Autodesk Inventor part; units mm, degrees
ref_plane "YZ Plane" through (0, 0, 0) normal (1, 0, 0) x (0, 1, 0)
ref_plane "XZ Plane" through (0, 0, 0) normal (0, 1, 0) x (-1, 0, 0)
ref_plane "XY Plane" through (0, 0, 0) normal (0, 0, 1) x (1, 0, 0)
sketch "Sketch1" plane through (0, 0, 0) normal (0, 0, 1) x (1, 0, 0)
  line L0 (38.1, -12.7) -> (-38.1, -12.7)
  line L1 (-38.1, -12.7) -> (-38.1, 12.7)
  line L2 (-38.1, 12.7) -> (38.1, 12.7)
  line L3 (38.1, 12.7) -> (38.1, -12.7)
  line L4 (38.1, -12.7) -> (-38.1, 12.7) construction
  line L5 (-38.1, -12.7) -> (38.1, 12.7) construction
  circle A0 centre (31.75, 6.35) radius 1.5875
  circle A1 centre (31.75, -6.35) radius 1.5875
  circle A2 centre (25.4, 6.35) radius 1.5875
  circle A3 centre (25.4, -6.35) radius 1.5875
  line L6 (-38.1, 12.7) -> (-63.5, 12.7)
  line L7 (-63.5, 12.7) -> (-63.5, -50.8)
  line L8 (-63.5, -50.8) -> (-38.1, -50.8)
  line L9 (-38.1, -50.8) -> (-38.1, 12.7)
  circle A4 centre (-38.1, -29.845) radius 17.145
  point P0 (0, 0)
  point P1 (-38.1, -46.99)
  dimension "d0" = 76.2
  dimension "d1" = 25.4
  dimension "d2" = 3.175
  dimension "d3" = 6.35
  dimension "d4" = 6.35
  dimension "d5" = 3.175
  dimension "d6" = 6.35
  dimension "d7" = 6.35
  dimension "d8" = 3.175
  dimension "d9" = 6.35
  dimension "d10" = 6.35
  dimension "d13" = 3.175
  dimension "d14" = 6.35
  dimension "d15" = 6.35
  dimension "d16" = 25.4
  dimension "d17" = 63.5
  dimension "d18" = 34.29
  dimension "d19" = 17.145
extrude "Extrusion1" add sketch "Sketch1" along normal blind 3.175 contours L0 L1 L2 L3 | A4 L9 L8 L7 L6 L1
fillet "Fillet1" radius 3.175 4 edges at (-38.1, -50.8, 1.5875) (-38.1, -46.99, 1.5875) (-63.5, -50.8, 1.5875) (-63.5, 12.7, 1.5875)
properties part number "Climb_Hooks_2"
Here's how the part is built. I have some questions about the finished solid (model axes, mm). Coordinates: 2 decimals unless noted, no trailing zeros. Order: outer loops, then holes, each group sorted by start corner. A loop starts at its lowest first (then second) coordinate and runs counter-clockwise, first axis right, second up. Notation, with made-up numbers: (34, 35.5) - (80, 35.5) arc R16 ccw to (80, 55.5) - close; hole circle Ø10 at (-6.75, 24). An arc over 180 degrees is marked (long way). One line per question, with ' | ' between items. Start each with the question number.
1. If we section it at B-B (x = 31.75): Write out the boundary of the cut face in (y, z) (1 decimal), and give its area (3 significant figures).
2. If we section it at A-A (y = 6.35): Write out the boundary of the cut face in (x, z) (1 decimal).
3. If we section it at C-C (z = 2.1): Give the number of separate pieces and of enclosed holes in the cut face, and give its area (3 significant figures).
4. Please list where these lines run through material, in increasing order: line 1 along Y through (x, z) = (32, 1.2); line 2 along X through (y, z) = (-5, 1.3); line 3 along Y through (x, z) = (33, 2.1). Write a range as [from, to].
5. I'm going to push a flat-ended pin straight in: pin 1 Ø1 at (x, z) = (-37.5, 0.5) entering from -Y. Where does the tip first touch, or does it pass through?
6. If we section it at D-D (x = -17): Write out the boundary of the cut face in (y, z) (3 decimals).
7. If we mould it in two halves opening along Y, with no side actions, what happens to faces 1 (the cylindrical face through (26.866, 6.958, 1.565)), 2 (the flat face through (-25, -4, 0)), 3 (the flat face through (-12, 12.7, 2)), 4 (the flat face through (1, -12.7, 2))? For each: released by +Y, released by -Y, zero draft, split by the parting line, or undercut.
Model answer:
1) outline: (-12.7, 0) - (-7.9, 0) - (-7.9, 3.2) - (-12.7, 3.2) - close; (-4.8, 0) - (4.8, 0) - (4.8, 3.2) - (-4.8, 3.2) - close; (7.9, 0) - (12.7, 0) - (12.7, 3.2) - (7.9, 3.2) - close | area: 60.5 mm²
2) outline: (-63.5, 0) - (23.8, 0) - (23.8, 3.2) - (-63.5, 3.2) - close; (27, 0) - (30.2, 0) - (30.2, 3.2) - (27, 3.2) - close; (33.3, 0) - (38.1, 0) - (38.1, 3.2) - (33.3, 3.2) - close
3) separate pieces: 1 | enclosed holes: 4 | area: 3,020 mm²
4) line 1: y = [-12.7, -7.92], [-4.78, 4.78], [7.92, 12.7] | line 2: x = [-63.5, 24.56], [26.24, 30.91], [32.59, 38.1] | line 3: y = [-12.7, -7.33], [-5.37, 5.37], [7.33, 12.7]
5) pin 1: stops at y = -12.7
6) outline: (-12.7, 0) - (12.7, 0) - (12.7, 3.175) - (-12.7, 3.175) - close
7) face 1: undercut | face 2: zero draft | face 3: released by +Y | face 4: released by -Y
